The figure shows three views and two pictorial views of one solid part (mm, origin at its lowest corner). Answer the questions. A direction names the side the tool comes from. Round coordinates to 2 decimals unless told otherwise and drop trailing zeros. Write each loop counter-clockwise with the first axis right and the second up, starting at its lowest first coordinate (ties: lowest second). Pieces come first, ordered by that corner, then holes. Notation, with made-up numbers: M 84,82.5 L 140,82.5 A36 cw 140,116.5 Z; hole C 56,84.25 d8. An arc over 180 degrees is marked long. Answer in a Markdown table with one row per item.
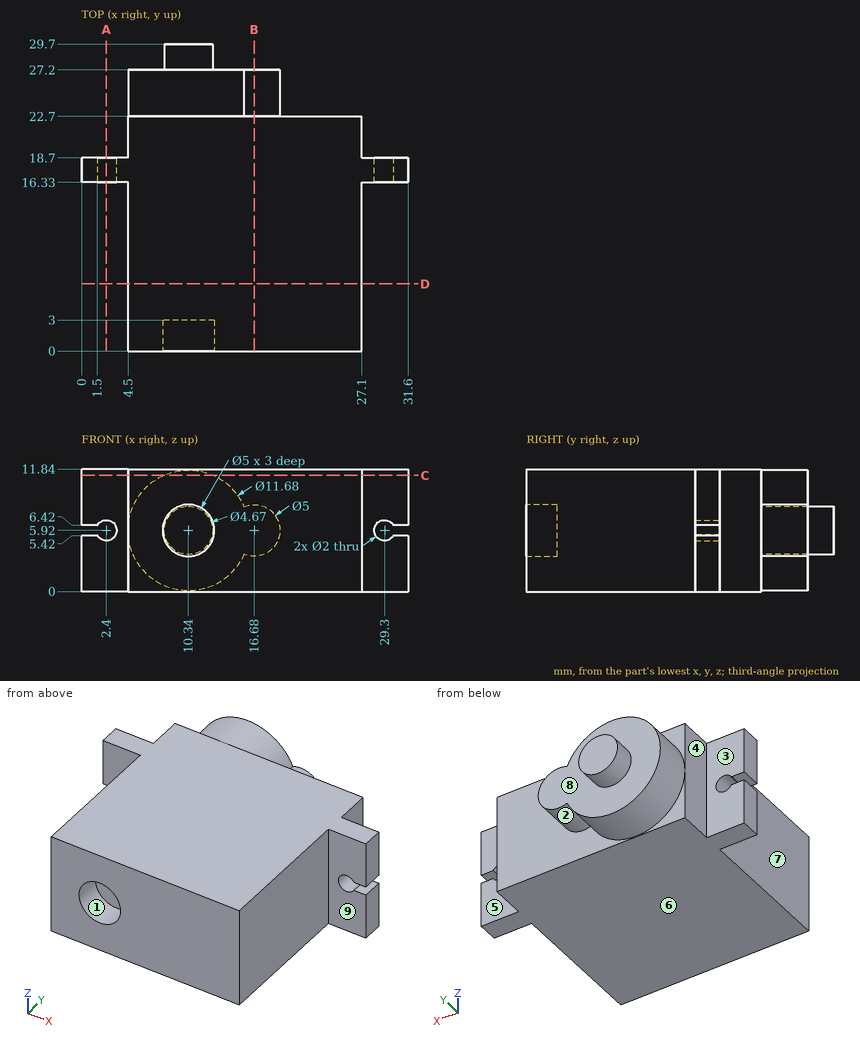
1. Consider line 1 along Z through (x, y) = (2.4, 17.4); line 2 along Z through (x, y) = (10.34, 1.85); line 3 along X through (y, z) = (9.75, 7.5). Determine where each line is inside the solid, lowest interval first. Write a range as from..to.
Calculated:
| item | result |
|---|---|
| line 1 | z = 0..4.92, 6.92..11.84 |
| line 2 | z = 0..3.42, 8.42..11.84 |
| line 3 | x = 4.5..27.1 |
2. The part is cut by section C-C (z = 11.25). Determine the outline of the cut face in (x, y).
Calculated:
| item | result |
|---|---|
| outline | M 0,16.33 L 4.5,16.33 L 4.5,0 L 27.1,0 L 27.1,16.33 L 31.6,16.33 L 31.6,18.7 L 27.1,18.7 L 27.1,22.7 L 12.73,22.7 L 12.73,27.2 L 7.95,27.2 L 7.95,22.7 L 4.5,22.7 L 4.5,18.7 L 0,18.7 Z |
3. The part is cut by section A-A (x = 2.4). Determine the outline of the cut face in (y, z).
Calculated:
| item | result |
|---|---|
| outline | M 16.33,0 L 18.7,0 L 18.7,4.92 L 16.33,4.92 Z; M 16.33,6.92 L 18.7,6.92 L 18.7,11.84 L 16.33,11.84 Z |
4. A tool of negligible diameter and unlimited length cuts with its end or side. For the marked faces 5, 6, 7, 8 and 9, from which of +Z, -Z, +X, -X, +Y, -Y can it reach the whole face along a straight path? Write none if from no direction.
Calculated:
| item | result |
|---|---|
| face 5 | +Z, -Z, +X, +Y |
| face 6 | -Z, +X, -X, +Y, -Y |
| face 7 | +Z, -Z, -X, -Y |
| face 8 | +Y |
| face 9 | +Z, -Z, +X, -Y |
5. Given pin 1 (3 mm diameter, centred on y = 20.5, z = 4, fed in from +X); pin 2 (5 mm diameter, centred on x = 1.5, z = 3.5, fed in from -Y); pin 3 (2 mm diameter, centred on x = 29, z = 3.5, fed in from +Y); pin 4 (1.8 mm diameter, centred on x = 29.3, z = 5.92, fed in from +Y), each flat-ended and moving along its own axis, determine where each tip first touches the part or whether it passes through.
Calculated:
| item | result |
|---|---|
| pin 1 | stops at x = 27.1 |
| pin 2 | stops at y = 16.33 |
| pin 3 | stops at y = 18.7 |
| pin 4 | passes through |
6. The part is cut by section B-B (x = 16.68). Determine the outline of the cut face in (y, z).
Calculated:
| item | result |
|---|---|
| outline | M 0,0 L 22.7,0 L 22.7,3.42 L 27.2,3.42 L 27.2,8.42 L 22.7,8.42 L 22.7,11.84 L 0,11.84 Z |
7. The part is cut by section D-D (y = 6.5). Determine the outline of the cut face in (x, z).
Calculated:
| item | result |
|---|---|
| outline | M 4.5,0 L 27.1,0 L 27.1,11.84 L 4.5,11.84 Z |
8. Determine the mould class of the marked faces 1, 2, 3 and 4 for opening direction X: released by +X, released by -X, zero draft, split by the parting line, or undercut.
Calculated:
| item | result |
|---|---|
| face 1 | undercut |
| face 2 | undercut |
| face 3 | zero draft |
| face 4 | released by -X |
